Can you work these out from the model? Positions are in its coordinate system, mm. Face numbers are marked on the shaded views. A direction names the side the tool comes from. Coordinates: 2 decimals unless noted, no trailing zeros. Order: outer loops, then holes, each group sorted by start corner. A loop starts at its lowest first (then second) coordinate and runs counter-clockwise, first axis right, second up. Notation, with made-up numbers: M -7,55.25 L 22,55.25 A13 cw 22,71.25 Z; hole C 77,30.25 d3. An arc over 180 degrees is marked long. Answer as CSV lines item,"result". Start each with the question number.
1. If we section it at B-B (y = -1.25): List the corners of the cut face in (x, z) for me, plus the area to 3 significant figures.
2. Will these pins go through, and if not, where does the flat tip stop? pin 1 (2 mm diameter, centred on x = 2.5, z = -17, fed in from +Y); pin 2 (4.5 mm diameter, centred on x = 2, z = 17, fed in from +Y).
3. If we section it at C-C (x = 0): List the corners of the cut face in (y, z) for me.
4. On a 3-axis mill with a long thin cutter (end or side, diameter ignored), from which of +Z, -Z, +X, -X, +Y, -Y can I reach the whole of each face in a straight line? I mean the marked faces 1 and 2. Say none if no direction works.
5. If we section it at D-D (y = -7.25): List the corners of the cut face in (x, z) for me.
6. I need wall thicknesses on line 1 along Z through (x, y) = (10, -5); line 2 along Z through (x, y) = (-2, -0.75); line 3 along X through (y, z) = (-6.5, 0). Which ranges of each line are inside material? Lowest first, please. Write a range as from..to.
7. If we mould it in two halves opening along X, with no side actions, what happens to the marked faces 3, 4, 5 and 6? For each: released by +X, released by -X, zero draft, split by the parting line, or undercut.
8. If we section it at A-A (z = 0): List the corners of the cut face in (x, y) for me.
```python
from build123d import *

# Parameters (mm, degrees)
SKETCH1_W           = 40.015172748
SKETCH1_H           = 40.015172748
BOSS_EXTRUDE1_DEPTH = 10
SKETCH2_R           = 8.75
CUT_EXTRUDE1_DEPTH  = 31.010115378
SKETCH3_W           = 22.4
SKETCH3_H           = 4.3
CUT_EXTRUDE3_DEPTH  = 6.7
SKETCH3_5_R         = 9.05
CUT_EXTRUDE4_DEPTH  = 9


with BuildPart() as part:
    # Sketch1 → Boss-Extrude1 (new body)
    with BuildSketch(Plane(origin=(0, 0, 0), x_dir=(1, 0, 0), z_dir=(0, 1, 0))):
        Rectangle(SKETCH1_W, SKETCH1_H)
    extrude(amount=-BOSS_EXTRUDE1_DEPTH)

    # Sketch2 → Cut-Extrude1 (cut, through all)
    with BuildSketch(Plane(origin=(0, 0, 0), x_dir=(1, 0, 0), z_dir=(0, 1, 0))):
        with Locations(Location((0, 0, 0), (0, 0, 270))):
            Circle(SKETCH2_R)
    extrude(amount=-CUT_EXTRUDE1_DEPTH, mode=Mode.SUBTRACT)

    # Sketch3 → Cut-Extrude3 (cut)
    with BuildSketch(Plane(origin=(0, 0, 0), x_dir=(1, 0, 0), z_dir=(0, 1, 0))):
        Polygon((11.2, 18.507586374), (0, 18.507586374), (-11.2, 18.507586374), (-11.2, 14.207586374), (0, 14.207586374), (11.2, 14.207586374), align=None)
        with Locations((0.1, -16.357586374)):
            Rectangle(SKETCH3_W, SKETCH3_H)
    extrude(amount=-CUT_EXTRUDE3_DEPTH, mode=Mode.SUBTRACT)

    # Sketch3<5> → Cut-Extrude4 (cut)
    with BuildSketch(Plane(origin=(0, 0, 0), x_dir=(1, 0, 0), z_dir=(0, 1, 0))):
        with Locations(Location((0, 0, 0), (0, 0, 270))):
            Circle(SKETCH3_5_R)
    extrude(amount=-CUT_EXTRUDE4_DEPTH, mode=Mode.SUBTRACT)


solid = part.part
```
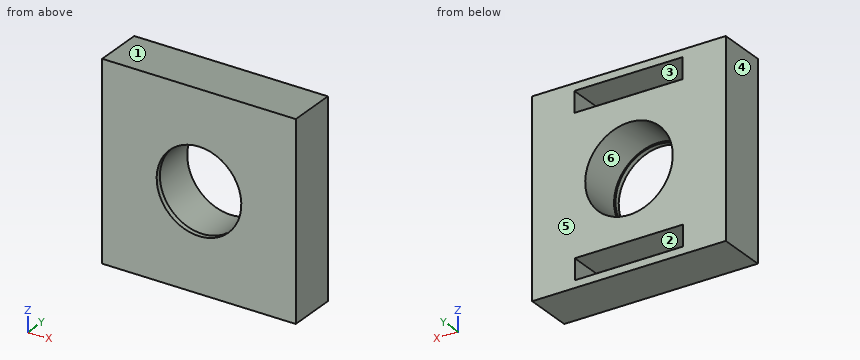
Solved:
1,outline,"M -20.01,-20.01 L 20.01,-20.01 L 20.01,20.01 L -20.01,20.01 Z; hole M -11.2,-18.51 L 11.2,-18.51 L 11.2,-14.21 L -11.2,-14.21 Z; hole M -11.1,14.21 L 11.3,14.21 L 11.3,18.51 L -11.1,18.51 Z; hole C 0,0 d18.1"
1,area,"1,150 mm²"
2,pin 1,"y = -6.7"
2,pin 2,"y = 0"
3,outline,"M -10,-20.01 L 0,-20.01 L 0,-18.51 L -6.7,-18.51 L -6.7,-14.21 L 0,-14.21 L 0,-9.05 L -9,-9.05 L -9,-8.75 L -10,-8.75 Z; M -10,8.75 L -9,8.75 L -9,9.05 L 0,9.05 L 0,14.21 L -6.7,14.21 L -6.7,18.51 L 0,18.51 L 0,20.01 L -10,20.01 Z"
4,face 1,"+Z, +X, -X, +Y, -Y"
4,face 2,"+Y"
5,outline,"M -20.01,-20.01 L 20.01,-20.01 L 20.01,20.01 L -20.01,20.01 Z; hole C 0,0 d18.1"
6,line 1,"-20.01..-18.51, -14.21..14.21, 18.51..20.01"
6,line 2,"-20.01..-18.51, -14.21..-8.83, 8.83..14.21, 18.51..20.01"
6,line 3,"-20.01..-9.05, 9.05..20.01"
7,face 3,"undercut"
7,face 4,"released by -X"
7,face 5,"zero draft"
7,face 6,"undercut"
8,outline,"M -20.01,-10 L -8.75,-10 L -8.75,-9 L -9.05,-9 L -9.05,0 L -20.01,0 Z; M 8.75,-10 L 20.01,-10 L 20.01,0 L 9.05,0 L 9.05,-9 L 8.75,-9 Z"
